Source: CAD feature listing. Evaluate the final solid. Frame: model axes, mm. A direction names the side the tool comes from. Round coordinates to 2 decimals unless told otherwise and drop trailing zeros. Loops run counter-clockwise (first coordinate to the right, second up) from the corner with the lowest first, then second, coordinate; pieces in that order, holes last. Notation, with made-up numbers: M 42,66.25 L 79,66.25 A6 ccw 79,71.25 Z; hole C -34.75,68.5 d5. An arc over 180 degrees is marked long. Answer as a JSON object with one key per item and string values.
from build123d import *

# Parameters (mm, degrees)
SKETCH1_R               = 17.5
BOSS_EXTRUDE1_DEPTH     = 10
SKETCH2_R               = 25
BOSS_EXTRUDE2_DEPTH     = 10
SKETCH3_R               = 17
BOSS_EXTRUDE3_DEPTH     = 5
SKETCH4_R               = 15
CUT_EXTRUDE1_DEPTH      = 1
CUT_EXTRUDE1_DEPTH_BACK = 26
FILLET1_R               = 1


with BuildPart() as part:
    # Sketch1 → Boss-Extrude1 (new body)
    with BuildSketch(Plane.XY):
        Circle(SKETCH1_R)
    extrude(amount=BOSS_EXTRUDE1_DEPTH)

    # Sketch2 → Boss-Extrude2 (add)
    with BuildSketch(Plane.XY.offset(10)):
        Circle(SKETCH2_R)
    extrude(amount=BOSS_EXTRUDE2_DEPTH)

    # Sketch3 → Boss-Extrude3 (add)
    with BuildSketch(Plane.XY.offset(20)):
        Circle(SKETCH3_R)
    extrude(amount=BOSS_EXTRUDE3_DEPTH)

    # Sketch4 → Cut-Extrude1 (cut, two sides)
    with BuildSketch(Plane.XY.offset(25)) as cut_extrude1_sk:
        Circle(SKETCH4_R)
    extrude(amount=CUT_EXTRUDE1_DEPTH, mode=Mode.SUBTRACT)
    extrude(cut_extrude1_sk.sketch, amount=-CUT_EXTRUDE1_DEPTH_BACK, mode=Mode.SUBTRACT)

    # Fillet1
    fillet1_edges = [part.edges().sort_by_distance(p)[0] for p in [
        (-25, 0, 10),
        (-25, 0, 20),
    ]]
    fillet(fillet1_edges, radius=FILLET1_R)


solid = part.part
Item 1: Section D-D on z = 14.75. Return the cut outline in (x, y).
Answer sheet:
{"outline": "C 0,0 d50; hole C 0,0 d30"}
Item 2: Section A-A on y = 0. Return the cut outline in (x, z).
Answer sheet:
{"outline": "M -25,11 A1 ccw -24,10 L -17.5,10 L -17.5,0 L -15,0 L -15,25 L -17,25 L -17,20 L -24,20 A1 ccw -25,19 Z; M 15,0 L 17.5,0 L 17.5,10 L 24,10 A1 ccw 25,11 L 25,19 A1 ccw 24,20 L 17,20 L 17,25 L 15,25 Z"}
Item 3: Pull-direction query (X, two-part tool) for faces 1 (the cylindrical face through (9.139, 14.334, 22.465)), 2 (the flat face through (6, -14, 25)), 3 (the cylindrical face through (-14.985, 0.66, 12.675)); classes: pulls with the +X half, pulls with the -X half, needs draft (parallel to the pull), parting line crosses it, or undercut.
Answer sheet:
{"face 1": "parting line crosses it", "face 2": "needs draft", "face 3": "undercut"}
Item 4: Contact query for flat-ended pins moving along their axis: pin 1 Ø12 at (x, z) = (-4, 18.5) entering from +Y; pin 2 Ø10 at (y, z) = (12, 18.5) entering from +X; pin 3 Ø12 at (x, y) = (-5.5, 19.5) entering from -Z; pin 4 Ø4 at (x, y) = (16, 13.5) entering from +Z. Output: stop coordinate, or through.
Answer sheet:
{"pin 1": "stops at y = 25", "pin 2": "stops at x = 24", "pin 3": "stops at z = 0", "pin 4": "stops at z = 20"}
Item 5: Section C-C on z = 23.25. Return the cut outline in (x, y).
Answer sheet:
{"outline": "C 0,0 d34; hole C 0,0 d30"}
Item 6: Access query for faces 4 (the flat face through (2, -18, 10)), 5 (the cylindrical face through (23.846, 7.509, 14.944)), 6 (the flat face through (-16.3, 5.7, 20)). Directions: +Z, -Z, +X, -X, +Y, -Y. A direction counts if a zero-diameter tool reaches every point of the face in a straight line with its end or side. Return the directions, or none.
Answer sheet:
{"face 4": "-Z", "face 5": "+Z, -Z", "face 6": "+Z"}
Item 7: Line query: probe 1 along Y at (x, z) = (0, 16.75); probe 2 along Y at (x, z) = (0, 8.5); probe 3 along Z at (x, y) = (-14, -10). Output: solid intervals per line, ascending. Write a range as from..to.
Answer sheet:
{"probe 1": "y = -25..-15, 15..25", "probe 2": "y = -17.5..-15, 15..17.5", "probe 3": "z = 0..20"}
